from build123d import *

# Parameters (mm, degrees)
F0_R      = 7.5
F0_R_2    = 10.5
F0_R_3    = 3.5
F1_DEPTH  = 42
F2_R      = 5
F2_R_2    = 3.5
F3_DEPTH  = 10
F4_R      = 3.5
F5_DEPTH  = 21
F6_R      = 16
F7_DEPTH  = 250
F8_R      = 2
F9_DEPTH  = 25
F10_R     = 7.5
F11_DEPTH = 15
F12_R     = 2
F13_DEPTH = 25
F14_R     = 16
F15_DEPTH = 20
F16_SIZE  = 2
F12_R_2   = 3.5
F17_DEPTH = 10


with BuildPart() as f1:
    # F0 (on Right) → F1 (new body)
    with BuildSketch(Plane.YZ):
        Polygon((112.5, 74.2), (112.5, 116.2), (35.5, 116.2), (-11.89577, 55.225982), (48.724809, -7.845921), align=None)
        with Locations((56.5, 95.2)):
            Circle(F0_R, mode=Mode.SUBTRACT)
        with Locations((91.5, 95.2)):
            Circle(F0_R_2, mode=Mode.SUBTRACT)
        Polygon((48.724809, -7.845921), (-11.89577, 55.225982), (-48.724809, 7.845921), (11.89577, -55.225982), align=None)
        with Locations((-10, -10)):
            Circle(F0_R_3, mode=Mode.SUBTRACT)
        with Locations((10, -10)):
            Circle(F0_R_3, mode=Mode.SUBTRACT)
        with Locations((-10, 10)):
            Circle(F0_R_3, mode=Mode.SUBTRACT)
        with Locations((10, 10)):
            Circle(F0_R_3, mode=Mode.SUBTRACT)
        Polygon((11.89577, -55.225982), (-48.724809, 7.845921), (-112.5, -74.2), (-112.5, -116.2), (-35.5, -116.2), align=None)
    extrude(amount=-F1_DEPTH)

    # F2 (on face) → F3 (cut)
    with BuildSketch(Plane(origin=(-42, 0, 0), x_dir=(0, -1, 0), z_dir=(-1, 0, 0))):
        with Locations((-10, 10)):
            Circle(F2_R)
        with Locations((-10, 10)):
            Circle(F2_R_2, mode=Mode.SUBTRACT)
        with Locations((-10, -10)):
            Circle(F2_R)
        with Locations((-10, -10)):
            Circle(F2_R_2, mode=Mode.SUBTRACT)
        with Locations((10, 10)):
            Circle(F2_R)
        with Locations((10, 10)):
            Circle(F2_R_2, mode=Mode.SUBTRACT)
        with Locations((10, -10)):
            Circle(F2_R)
        with Locations((10, -10)):
            Circle(F2_R_2, mode=Mode.SUBTRACT)
    extrude(amount=-F3_DEPTH, mode=Mode.SUBTRACT)

    # F4 (on face) → F5 (cut)
    with BuildSketch(Plane.YZ):
        Polygon((11.138655, -56.2), (98.508403, 56.2), (-11.138655, 56.2), (-98.508403, -56.2), align=None)
        with Locations((-10, -10)):
            Circle(F4_R, mode=Mode.SUBTRACT)
        with Locations((10, -10)):
            Circle(F4_R, mode=Mode.SUBTRACT)
        with Locations((-10, 10)):
            Circle(F4_R, mode=Mode.SUBTRACT)
        with Locations((10, 10)):
            Circle(F4_R, mode=Mode.SUBTRACT)
    extrude(amount=-F5_DEPTH, mode=Mode.SUBTRACT)

    # F6 (on face) → F7 (cut)
    with BuildSketch(Plane(origin=(0, 112.5, 0), x_dir=(-1, 0, 0), z_dir=(0, 1, 0))):
        with Locations((21, -95.2)):
            Circle(F6_R)
    extrude(amount=-F7_DEPTH, mode=Mode.SUBTRACT)

    # F8 (on face) → F9 (cut)
    with BuildSketch(Plane(origin=(0, 0, -116.2), x_dir=(1, 0, 0), z_dir=(0, 0, -1))):
        with Locations((-21, 49.5)):
            Circle(F8_R)
        with Locations((-21, 91.5)):
            Circle(F8_R)
    extrude(amount=-F9_DEPTH, mode=Mode.SUBTRACT)

    # F10 (on face) → F11 (cut)
    with BuildSketch(Plane(origin=(-42, 0, 0), x_dir=(0, -1, 0), z_dir=(-1, 0, 0))):
        Polygon((-35.5, 116.2), (-76, 116.2), (-76, 74.389189), (-3, 74.389189), align=None)
        with Locations((-56.5, 95.2)):
            Circle(F10_R, mode=Mode.SUBTRACT)
        Polygon((-3, 116.389189), (-76, 116.389189), (-76, 116.2), (-35.5, 116.2), (-3, 74.389189), align=None)
    extrude(amount=-F11_DEPTH, mode=Mode.SUBTRACT)

    # F12 (on face) → F13 (cut)
    with BuildSketch(Plane.XY.offset(116.2)):
        with Locations((-21, 91.5)):
            Circle(F12_R)
        with Locations((-15, 56.5)):
            Circle(F12_R)
        with Locations((-5, 56.5)):
            Circle(F12_R)
    extrude(amount=-F13_DEPTH, mode=Mode.SUBTRACT)

    # F14 (on face) → F15 (cut)
    with BuildSketch(Plane.YZ):
        with Locations((56.5, 95.2)):
            Circle(F14_R)
    extrude(amount=-F15_DEPTH, mode=Mode.SUBTRACT)

    # F16
    f16_edges = [f1.edges().sort_by_distance(p)[0] for p in [
        (0, 43.684874, 56.2),
        (0, -43.684874, -56.2),
        (-42, -74, -116.2),
        (0, -74, -116.2),
        (0, 74, 116.2),
        (-21, -54.823529, 0),
        (-21, 54.823529, 0),
        (-42, 39.5, 74.389189),
        (-42, 76, 95.294595),
    ]]
    chamfer(f16_edges, length=F16_SIZE)

    # F12 (on face) → F17 (cut)
    with BuildSketch(Plane.XY.offset(116.2)):
        with Locations((-22, 71.5)):
            Circle(F12_R_2)
        with Locations((-22, 41.5)):
            Circle(F12_R_2)
    extrude(amount=-F17_DEPTH, mode=Mode.SUBTRACT)


solid = f1.part
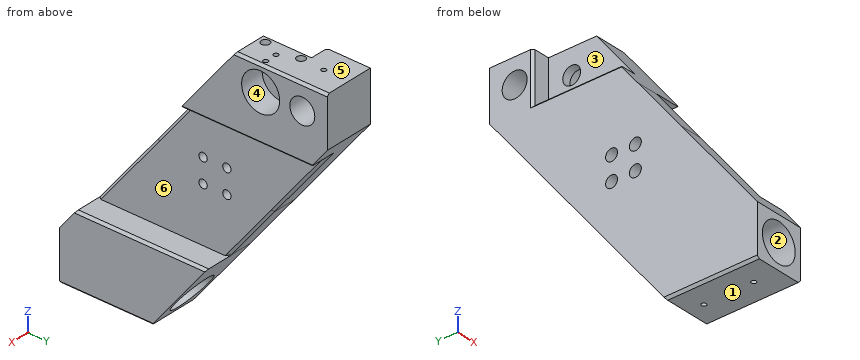
Work out the finished part from the listing and answer in its coordinate system (mm). Face numbers are marked on the shaded views. A direction names the side the tool comes from. Give positions to 0.01 mm unless a question says otherwise; leave off trailing zeros. Order: outer loops, then holes, each group sorted by start corner. A loop starts at its lowest first (then second) coordinate and runs counter-clockwise, first axis right, second up. Notation, with made-up numbers: (-22.75, 70.5) -> (32.25, 70.5) arc R21 cw to (32.25, 104.5) -> close; hole circle Ø10 at (65, 1). An arc over 180 degrees is marked (long way). Answer as a JSON object with one key per item and string values. Group by question number.
1. Section B-B on z = 35.5 is taken. Determine the outline of the cut face in (x, y), plus the area to 3 significant figures.
2. Consider line 1 along X through (y, z) = (56.5, 113.5); line 2 along Y through (x, z) = (-27, 10); line 3 along Z through (x, y) = (-39, 6.5). Determine where each line is inside the solid, lowest interval first. Write a range as [from, to].
3. Flat-ended cylindrical pins translate along their axes: pin 1 Ø9 at (y, z) = (-10, 10) entering from -X; pin 2 Ø6.5 at (x, y) = (-9, 43) entering from -Z; pin 3 Ø10 at (y, z) = (22.5, 78) entering from -X. Find the tip coordinate at first contact, or state that the pin passes through.
4. Section C-C on z = 63 is taken. Determine the outline of the cut face in (x, y).
5. A tool of negligible diameter and unlimited length cuts with its end or side. For the marked faces 4, 5 and 6, from which of +Z, -Z, +X, -X, +Y, -Y can it reach the whole face along a straight path? Write none if from no direction.
6. The mould has two halves that part along Z. Classify the marked faces 1, 2 and 3: released by +Z, released by -Z, zero draft, split by the parting line, or undercut.
7. Section A-A on y = -86 is taken. Determine the outline of the cut face in (x, z).
Result sheet:
{
 "1": {"outline": "(-42, -27.23) -> (-23, -27.23) -> (-21, -24.7) -> (-21, 79.88) -> (-23, 82.42) -> (-42, 82.42) -> close", "area": "2,300 mm^2"},
 "2": {"line 1": "x = [-27, -17], [-13, -7], [-3, 0]", "line 2": "y = [-47.05, -13.5], [-6.5, 6.5], [13.5, 62.6]", "line 3": "z = [-62.17, -13.57], [-6.43, 6.43], [13.57, 74.39]"},
 "3": {"pin 1": "stops at x = -32", "pin 2": "stops at z = 56.2", "pin 3": "stops at x = -41.39"},
 "4": {"outline": "(-42, -5.85) -> (0, -5.85) -> (0, 103.79) -> (-42, 103.79) -> close"},
 "5": {"face 4": "+X", "face 5": "+Z, +X, -X, +Y, -Y", "face 6": "+X, +Y, -Y"},
 "6": {"face 1": "released by -Z", "face 2": "undercut", "face 3": "zero draft"},
 "7": {"outline": "(-42, -114.2) -> (-40, -116.2) -> (-2, -116.2) -> (0, -114.2) -> (0, -58.2) -> (-2, -56.2) -> (-21, -56.2) -> (-21, -43.37) -> (-23, -40.11) -> (-42, -40.11) -> close; hole circle Ø32 at (-21, -95.2)"}
}
